```python
from build123d import *

# Parameters (mm, degrees)
SKETCH1_R           = 1.5
SKETCH1_W           = 14
SKETCH1_H           = 15.525
SKETCH1_W_2         = 46.75
SKETCH1_H_2         = 20.3
BOSS_EXTRUDE1_DEPTH = 3.75
CUT_EXTRUDE1_DEPTH  = 118.232216135
SKETCH3_W           = 99.3
SKETCH3_H           = 62.2
BOSS_EXTRUDE2_DEPTH = 3
SKETCH4_R           = 1.5
CUT_EXTRUDE2_DEPTH  = 4.75
FILLET1_R           = 0.5


with BuildPart() as part:
    # Sketch1 → Boss-Extrude1 (new body)
    with BuildSketch(Plane(origin=(0, 0, 0), x_dir=(1, 0, 0), z_dir=(0, 1, 0))):
        Polygon((0, 62.2), (0, 0), (35, 0), (35, 3), (4.525, 3), (4.525, 18.525), (75.675, 18.525), (75.675, 3), (45, 3), (45, 0), (99.3, 0), (99.3, 62.2), align=None)
        with Locations(Location((10, 25, 0), (0, 0, 270))):
            Circle(SKETCH1_R, mode=Mode.SUBTRACT)
        with Locations(Location((89.25, 10, 0), (0, 0, 270))):
            Circle(SKETCH1_R, mode=Mode.SUBTRACT)
        with Locations((87.725, 29.8125)):
            Rectangle(SKETCH1_W, SKETCH1_H, mode=Mode.SUBTRACT)
        with Locations(Location((25, 47.15, 0), (0, 0, 270))):
            Circle(SKETCH1_R, mode=Mode.SUBTRACT)
        with Locations(Location((74.25, 37.15, 0), (0, 0, 270))):
            Circle(SKETCH1_R, mode=Mode.SUBTRACT)
        with Locations((68.675, 50.3)):
            Rectangle(SKETCH1_W_2, SKETCH1_H_2, mode=Mode.SUBTRACT)
    extrude(amount=BOSS_EXTRUDE1_DEPTH)

    # Sketch2 → Cut-Extrude1 (cut, through all)
    with BuildSketch(Plane.XZ):
        Polygon((19, -18.525), (19, -28), (32, -28), (32, -50), (45.3, -50), (45.3, -40.15), (52, -40.15), (52, -30), (68, -30), (68, -18.525), align=None)
    extrude(amount=-CUT_EXTRUDE1_DEPTH, mode=Mode.SUBTRACT)

    # Sketch3 → Boss-Extrude2 (add)
    with BuildSketch(Plane(origin=(0, 3.75, 0), x_dir=(1, 0, 0), z_dir=(0, 1, 0))):
        with Locations((49.65, 31.1)):
            Rectangle(SKETCH3_W, SKETCH3_H)
    extrude(amount=BOSS_EXTRUDE2_DEPTH)

    # Sketch4 → Cut-Extrude2 (cut)
    with BuildSketch(Plane.XZ):
        with Locations(Location((89.25, -10, 0), (0, 0, 90))):
            Circle(SKETCH4_R)
        with Locations(Location((74.25, -37.15, 0), (0, 0, 90))):
            Circle(SKETCH4_R)
        with Locations(Location((25, -47.15, 0), (0, 0, 90))):
            Circle(SKETCH4_R)
        with Locations(Location((10, -25, 0), (0, 0, 90))):
            Circle(SKETCH4_R)
    extrude(amount=-CUT_EXTRUDE2_DEPTH, mode=Mode.SUBTRACT)

    # Fillet1
    fillet1_edges = [part.edges().sort_by_distance(p)[0] for p in [
        (0, 6.75, -31.1),
        (49.65, 6.75, 0),
        (99.3, 6.75, -31.1),
        (49.65, 6.75, -62.2),
        (0, 3.375, 0),
        (0, 3.375, -62.2),
        (99.3, 3.375, -62.2),
        (99.3, 3.375, 0),
        (35, 3.75, -1.5),
        (45, 3.75, -1.5),
    ]]
    fillet(fillet1_edges, radius=FILLET1_R)


solid = part.part
```
Work out the finished part from the listing and answer in its coordinate system (mm). A direction names the side the tool comes from. Give positions to 0.01 mm unless a question says otherwise; leave off trailing zeros. Loops run counter-clockwise (first coordinate to the right, second up) from the corner with the lowest first, then second, coordinate; pieces in that order, holes last. Notation, with made-up numbers: (55.25, 41.25) -> (94.25, 41.25) arc R24 ccw to (94.25, 52.25) -> close; hole circle Ø8 at (55.5, 18). An arc over 180 degrees is marked (long way). Write item = value, one per line. Start each with the question number.
(1) Find section B-B on x = 77.5. Give the vertices of the cut face in (y, z), and give its area (3 significant figures).
(2) Find section A-A on z = -32. Give the vertices of the cut face in (x, y) (3 decimals).
(3) The mould has two halves that part along Z. Classify faces 1 (the flat face through (49, 3, -62.2)), 2 (the flat face through (12, 2, -18.525)), 3 (the flat face through (45, 2, -2)): +Z half, -Z half, draft (parallel to the pull), parting line (faces both ways), or undercut.
(4) Which of the six approach directions +Z, -Z, +X, -X, +Y, -Y give full straight-line access (tool end or side, diameter ignored) to faces 4 (the flat face through (0, 3, -31)), 5 (the flat face through (20, 2, -3))?
(5) Find the intervals of material crossed by probe 1 along Z at (x, y) = (82.5, 3) (3 decimals); probe 2 along X at (y, z) = (1.75, -33.5) (3 decimals); probe 3 along X at (y, z) = (1.35, -37.15) (3 decimals), in increasing order. Write a range as from..to.
(6) Find section C-C on z = -4. Give the vertices of the cut face in (x, y) (3 decimals).
(7) Find section D-D on x = 62. Give the vertices of the cut face in (y, z), and give its area (3 significant figures).
(8) Given pin 1 Ø1.8 at (x, z) = (89.25, -10) entering from -Y, flat-ended and moving along its own axis, determine where the tip first touches the part or whether it passes through.
From the geometry:
q1.outline = (0, -62.2) -> (6.25, -62.2) arc R0.5 ccw to (6.75, -61.7) -> (6.75, -0.5) arc R0.5 ccw to (6.25, 0) -> (0, 0) -> (0, -40.15) -> (3.75, -40.15) -> (3.75, -60.45) -> (0, -60.45) -> close
q1.area = 344 mm^2
q2.outline = (0, 0) -> (32, 0) -> (32, 3.75) -> (52, 3.75) -> (52, 0) -> (80.725, 0) -> (80.725, 3.75) -> (94.725, 3.75) -> (94.725, 0) -> (99.3, 0) -> (99.3, 6.25) arc R0.5 ccw to (98.8, 6.75) -> (0.5, 6.75) arc R0.5 ccw to (0, 6.25) -> close
q3.face_1 = -Z half
q3.face_2 = undercut
q3.face_3 = draft
q4.face_4 = +Z, -Z, -X, +Y, -Y
q4.face_5 = -Y
q5.probe_1 = -62.2..-60.45, -40.15..-37.575, -22.05..0
q5.probe_2 = 0..32, 52..80.725, 94.725..99.3
q5.probe_3 = 0..32, 52..72.75, 75.75..80.725, 94.725..99.3
q6.outline = (0, 0) -> (4.525, 0) -> (4.525, 3.75) -> (75.675, 3.75) -> (75.675, 0) -> (99.3, 0) -> (99.3, 6.25) arc R0.5 ccw to (98.8, 6.75) -> (0.5, 6.75) arc R0.5 ccw to (0, 6.25) -> close
q7.outline = (0, -62.2) -> (6.25, -62.2) arc R0.5 ccw to (6.75, -61.7) -> (6.75, -0.5) arc R0.5 ccw to (6.25, 0) -> (0, 0) -> (0, -3) -> (3.75, -3) -> (3.75, -30) -> (0, -30) -> (0, -40.15) -> (3.75, -40.15) -> (3.75, -60.45) -> (0, -60.45) -> close
q7.area = 242 mm^2
q8.pin_1 = 4.75
